CAD build for the part. Positions are in the model's coordinates, mm. Face numbers are marked on the shaded views. A direction names the side the tool comes from. Round coordinates to 2 decimals unless told otherwise and drop trailing zeros. Loops run counter-clockwise (first coordinate to the right, second up) from the corner with the lowest first, then second, coordinate; pieces in that order, holes last.
```python
from build123d import *

# Parameters (mm, degrees)
F0_R     = 1.05
F1_DEPTH = 6


with BuildPart() as f1:
    # F0 (on Top) → F1 (new body)
    with BuildSketch(Plane.XY):
        with BuildLine():
            Line((-2.298571, -10.070698), (-0.453154, -14.028208))
            ThreePointArc((-0.453154, -14.028208), (0, -14.316899), (0.453154, -14.028208))
            Line((0.453154, -14.028208), (2.298571, -10.070698))
            Line((2.298571, -10.070698), (5.678334, -12.835595))
            ThreePointArc((5.678334, -12.835595), (6.21187, -12.89908), (6.494889, -12.442363))
            Line((6.494889, -12.442363), (6.440453, -8.076073))
            Line((6.440453, -8.076073), (10.685158, -9.100735))
            ThreePointArc((10.685158, -9.100735), (11.193403, -8.926441), (11.250232, -8.392155))
            Line((11.250232, -8.392155), (9.306725, -4.481882))
            Line((9.306725, -4.481882), (13.575656, -3.563362))
            ThreePointArc((13.575656, -3.563362), (13.957945, -3.18581), (13.777328, -2.679778))
            Line((13.777328, -2.679778), (10.329685, 0))
            Line((10.329685, 0), (13.777328, 2.679778))
            ThreePointArc((13.777328, 2.679778), (13.957945, 3.18581), (13.575656, 3.563362))
            Line((13.575656, 3.563362), (9.306725, 4.481882))
            Line((9.306725, 4.481882), (11.250232, 8.392155))
            ThreePointArc((11.250232, 8.392155), (11.193403, 8.926441), (10.685158, 9.100735))
            Line((10.685158, 9.100735), (6.440453, 8.076073))
            Line((6.440453, 8.076073), (6.494889, 12.442363))
            ThreePointArc((6.494889, 12.442363), (6.21187, 12.89908), (5.678334, 12.835595))
            Line((5.678334, 12.835595), (2.298571, 10.070698))
            Line((2.298571, 10.070698), (0.453154, 14.028208))
            ThreePointArc((0.453154, 14.028208), (0, 14.316899), (-0.453154, 14.028208))
            Line((-0.453154, 14.028208), (-2.298571, 10.070698))
            Line((-2.298571, 10.070698), (-5.678334, 12.835595))
            ThreePointArc((-5.678334, 12.835595), (-6.21187, 12.89908), (-6.494889, 12.442363))
            Line((-6.494889, 12.442363), (-6.440453, 8.076073))
            Line((-6.440453, 8.076073), (-10.685158, 9.100735))
            ThreePointArc((-10.685158, 9.100735), (-11.193403, 8.926441), (-11.250232, 8.392155))
            Line((-11.250232, 8.392155), (-9.306725, 4.481882))
            Line((-9.306725, 4.481882), (-13.575656, 3.563362))
            ThreePointArc((-13.575656, 3.563362), (-13.957945, 3.18581), (-13.777328, 2.679778))
            Line((-13.777328, 2.679778), (-10.329685, 0))
            Line((-10.329685, 0), (-13.777328, -2.679778))
            ThreePointArc((-13.777328, -2.679778), (-13.957945, -3.18581), (-13.575656, -3.563362))
            Line((-13.575656, -3.563362), (-9.306725, -4.481882))
            Line((-9.306725, -4.481882), (-11.250232, -8.392155))
            ThreePointArc((-11.250232, -8.392155), (-11.193403, -8.926441), (-10.685158, -9.100735))
            Line((-10.685158, -9.100735), (-6.440453, -8.076073))
            Line((-6.440453, -8.076073), (-6.494889, -12.442363))
            ThreePointArc((-6.494889, -12.442363), (-6.21187, -12.89908), (-5.678334, -12.835595))
            Line((-5.678334, -12.835595), (-2.298571, -10.070698))
        make_face()
        Circle(F0_R, mode=Mode.SUBTRACT)
    extrude(amount=F1_DEPTH)


solid = f1.part
```
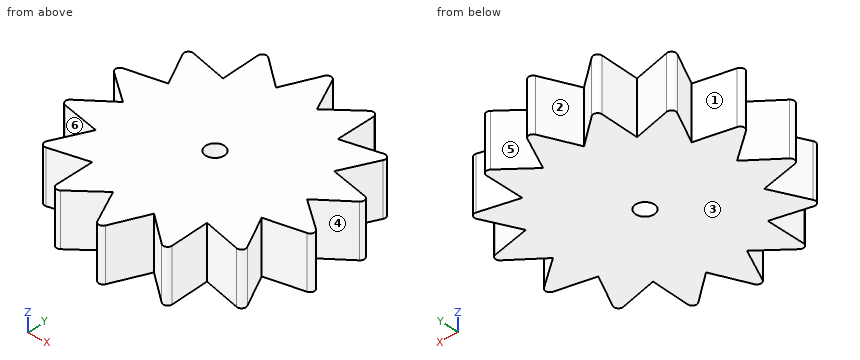
Item 1: Cut at B-B, the plane y = 11.75. Give the cut face in (x, z), plus the area to 3 significant figures.
Answers follow:
outline: (-6.49, 0) - (-4.35, 0) - (-4.35, 6) - (-6.49, 6) - close; (-1.52, 0) - (1.52, 0) - (1.52, 6) - (-1.52, 6) - close; (4.35, 0) - (6.49, 0) - (6.49, 6) - (4.35, 6) - close
area: 43.8 mm2
Item 2: Cut at D-D, the plane y = 5.5. Give the cut face in (x, z), plus the area to 3 significant figures.
Answers follow:
outline: (-9.81, 0) - (9.81, 0) - (9.81, 6) - (-9.81, 6) - close
area: 118 mm2
Item 3: Two-plate mould, pull along Y, no slides. Class the marked faces 1, 2 and 3: released by +Y, released by -Y, zero draft, split by the parting line, or undercut.
Answers follow:
face 1: undercut
face 2: released by +Y
face 3: zero draft
Item 4: Flat gauge pins, fed straight in: P1, Ø2, axis at y = -10.5, z = 2.5, coming from the -X side; P2, Ø1.5, axis at y = 7, z = 4, coming from the +X side. Where does each tip first touch, or does it go through?
Answers follow:
P1: stops at x = -6.48
P2: stops at x = 10.93
Item 5: 3-axis set-ups, long thin cutter, end or side, ignore diameter. For the marked faces 4, 5 and 6: which of +Z, -Z, +X, -X, +Y, -Y reach the whole face in a straight line?
Answers follow:
face 4: +Z, -Z, +X
face 5: +Z, -Z, +Y
face 6: +Z, -Z, -X
Item 6: Probe line 1 (Y direction, x = 0, z = 1.3); line 2 (X direction, y = 11.75, z = 2.65); line 3 (Y direction, x = 10, z = 3.9). List the from-to ranges inside material, lowest first.
Answers follow:
line 1: y = -14.32 to -1.05, 1.05 to 14.32
line 2: x = -6.49 to -4.35, -1.52 to 1.52, 4.35 to 6.49
line 3: y = -8.94 to -5.88, -4.33 to 4.33, 5.88 to 8.94
Item 7: Cut at A-A, the plane x = 0. Give the cut face in (y, z).
Answers follow:
outline: (-14.32, 0) - (-1.05, 0) - (-1.05, 6) - (-14.32, 6) - close; (1.05, 0) - (14.32, 0) - (14.32, 6) - (1.05, 6) - close
Item 8: Cut at C-C, the plane x = -7. Give the cut face in (y, z), plus the area to 3 significant figures.
Answers follow:
outline: (-8.21, 0) - (8.21, 0) - (8.21, 6) - (-8.21, 6) - close
area: 98.5 mm2
